```python
from build123d import *

# Parameters (mm, degrees)
SKETCH1_R           = 10
BOSS_EXTRUDE1_DEPTH = 11
SKETCH2_R           = 8.5
SKETCH2_R_2         = 6
CUT_EXTRUDE1_DEPTH  = 10
SKETCH3_R           = 5
CUT_EXTRUDE2_DEPTH  = 10


with BuildPart() as part:
    # Sketch1 → Boss-Extrude1 (new body)
    with BuildSketch(Plane(origin=(0, 0, 0), x_dir=(1, 0, 0), z_dir=(0, 1, 0))):
        with Locations((-45.043259766, 0)):
            Circle(SKETCH1_R)
    extrude(amount=BOSS_EXTRUDE1_DEPTH)

    # Sketch2 → Cut-Extrude1 (cut)
    with BuildSketch(Plane(origin=(0, 11, 0), x_dir=(1, 0, 0), z_dir=(0, 1, 0))):
        with Locations((-45.043259766, 0)):
            Circle(SKETCH2_R)
        with Locations((-45.043259766, 0)):
            Circle(SKETCH2_R_2, mode=Mode.SUBTRACT)
    extrude(amount=-CUT_EXTRUDE1_DEPTH, mode=Mode.SUBTRACT)

    # Sketch3 → Cut-Extrude2 (cut)
    with BuildSketch(Plane(origin=(0, 11, 0), x_dir=(1, 0, 0), z_dir=(0, 1, 0))):
        with Locations((-45.043259766, 0)):
            Circle(SKETCH3_R)
    extrude(amount=-CUT_EXTRUDE2_DEPTH, mode=Mode.SUBTRACT)


solid = part.part
```
Here's how the part is built. I have some questions about the finished solid (model axes, mm). A direction names the side the tool comes from. Round coordinates to 2 decimals unless told otherwise and drop trailing zeros. Write each loop counter-clockwise with the first axis right and the second up, starting at its lowest first coordinate (ties: lowest second). Pieces come first, ordered by that corner, then holes. Notation, with made-up numbers: M 48.5,34.25 L 75.5,34.25 A8 cw 75.5,39.25 Z; hole C -0.5,-27 d10. An arc over 180 degrees is marked long. Answer as CSV lines item,"result". Start each with the question number.
1. Suppose I cut it at C-C on x = -42.25. Write out the boundary of the cut face in (y, z).
2. I need wall thicknesses on probe 1 along X at (y, z) = (8.5, 0); probe 2 along Z at (x, y) = (-47.5, 4.5); probe 3 along Z at (x, y) = (-48, 5.75). Which ranges of each line are inside material? Lowest first, please.
3. Thinking about a two-plate mould opening in Z: for faces 3 (the cylindrical face through (-51.037, 6.07, -0.264)), 4 (the flat face through (-48.1, 11, 8.1)), 5 (the cylindrical face through (-52.979, 5.423, 6.085)), which applies, released by +Z, released by -Z, zero draft, split by the parting line, or undercut?
4. Suppose I cut it at B-B on y = 10. Write out the boundary of the cut face in (x, z).
5. Suppose I cut it at A-A on z = 0. Write out the boundary of the cut face in (x, y).
6. Suppose I cut it at D-D on z = 8. Write out the boundary of the cut face in (x, y), then the cut area to 3 significant figures.
7. On a 3-axis mill with a long thin cutter (end or side, diameter ignored), from which of +Z, -Z, +X, -X, +Y, -Y can I reach the whole of each face in a straight line? I mean faces 1 (the flat face through (-49, 11, -4)), 2 (the flat face through (-43, 1, -6)). Say none if no direction works.
8. I'm going to push flat-ended pins straight in: pin 1 Ø8 at (x, z) = (-45.04, 0) entering from +Y; pin 2 Ø1 at (x, y) = (-48, 1.5) entering from +Z; pin 3 Ø2 at (y, z) = (2.5, -3) entering from -X. Where does each tip first touch, or does it pass through?
Check result:
1,outline,"M 0,-9.6 L 11,-9.6 L 11,-8.03 L 1,-8.03 L 1,-5.31 L 11,-5.31 L 11,-4.15 L 1,-4.15 L 1,4.15 L 11,4.15 L 11,5.31 L 1,5.31 L 1,8.03 L 11,8.03 L 11,9.6 L 0,9.6 Z"
2,probe 1,"x = -55.04 to -53.54, -51.04 to -50.04, -40.04 to -39.04, -36.54 to -35.04"
2,probe 2,"z = -9.69 to -8.14, -5.47 to -4.35, 4.35 to 5.47, 8.14 to 9.69"
2,probe 3,"z = -9.55 to -7.97, -5.22 to -4.03, 4.03 to 5.22, 7.97 to 9.55"
3,face 3,"undercut"
3,face 4,"zero draft"
3,face 5,"split by the parting line"
4,outline,"C -45.04,0 d20; C -45.04,0 d12; hole C -45.04,0 d17; hole C -45.04,0 d10"
5,outline,"M -55.04,0 L -35.04,0 L -35.04,11 L -36.54,11 L -36.54,1 L -39.04,1 L -39.04,11 L -40.04,11 L -40.04,1 L -50.04,1 L -50.04,11 L -51.04,11 L -51.04,1 L -53.54,1 L -53.54,11 L -55.04,11 Z"
6,outline,"M -51.04,0 L -39.04,0 L -39.04,11 L -42.17,11 L -42.17,1 L -47.92,1 L -47.92,11 L -51.04,11 Z"
6,area,"74.6 mm2"
7,face 1,"+Z, -Z, +X, -X, +Y"
7,face 2,"+Y"
8,pin 1,"stops at y = 1"
8,pin 2,"stops at z = 9.69"
8,pin 3,"stops at x = -54.84"
